Verification items for the finished model (mm, model axes). Face numbers are marked on the shaded views. A direction names the side the tool comes from. Give positions to 0.01 mm unless a question says otherwise; leave off trailing zeros. Order: outer loops, then holes, each group sorted by start corner. A loop starts at its lowest first (then second) coordinate and runs counter-clockwise, first axis right, second up.
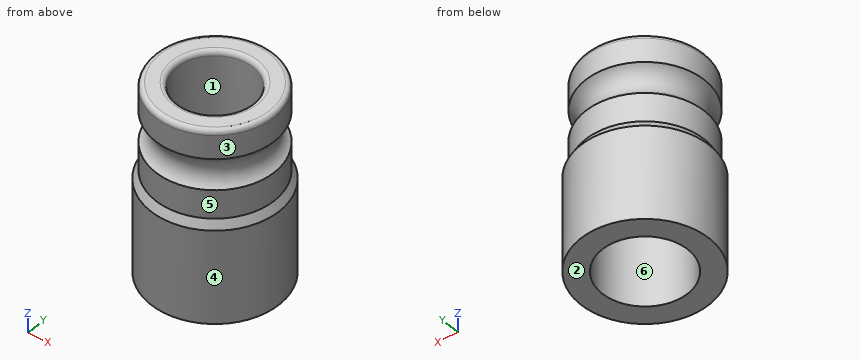
from build123d import *

# Parameters (mm, degrees)
F2_R     = 2
F3_R     = 18
F3_R_2   = 14
F4_DEPTH = 30


# Not quite as in the source:
# - a feature names something its author has since deleted; it is built from what else it names


with BuildPart() as f1:
    # F0 (on Front) → F1 (revolve)
    with BuildSketch(Plane.XZ):
        with BuildLine():
            Line((-14, -9.4360596032), (-16, 40.5639403968))
            Line((-16, 40.5639403968), (-25, 40.5639403968))
            Line((-25, 40.5639403968), (-25, 28.5639403968))
            ThreePointArc((-25, 28.5639403968), (-21.593316446, 22.014021006), (-25, 15.4641016151))
            Line((-25, 15.4641016151), (-25, 3.4641016151))
            Line((-25, 3.4641016151), (-27, 0))
            Line((-27, 0), (-27, -39.4360596032))
            Line((-27, -39.4360596032), (-18, -39.4360596032))
            Line((-18, -39.4360596032), (-14, -39.4360596032))
            Line((-14, -39.4360596032), (-14, -9.4360596032))
        make_face()
    revolve(axis=Axis((0, 0, -1.7232764512), (0, 0, -1)))

    # F2
    f2_edges = [f1.edges().sort_by_distance(p)[0] for p in [
        (16, 0, 40.56394),
        (25, 0, 40.56394),
    ]]
    fillet(f2_edges, radius=F2_R)

    # F3 (on face) → F4 (cut)
    with BuildSketch(Plane(origin=(0, 0, -39.4360596032), x_dir=(1, 0, 0), z_dir=(0, 0, -1))):
        Circle(F3_R)
        Circle(F3_R_2, mode=Mode.SUBTRACT)
    extrude(amount=-F4_DEPTH, mode=Mode.SUBTRACT)


solid = f1.part
(1) Set-up check for the marked faces 4, 5 and 6: record each of +Z, -Z, +X, -X, +Y, -Y from which the full face is reachable in a straight line by a thin tool's end or side.
Solved:
face 4: +Z, -Z
face 5: +Z
face 6: -Z
(2) Go/stop test with flat-tipped pins: pin 1 (1 mm diameter, centred on x = 4.5, z = -21.5, fed in from -Y); pin 2 (8 mm diameter, centred on x = -5.5, z = 28, fed in from -Y); pin 3 (11 mm diameter, centred on x = 3.5, y = 2, fed in from -Z); pin 4 (4 mm diameter, centred on x = 9, z = -0.5, fed in from +Y). Record where each tip stops, or that it passes through.
Solved:
pin 1: stops at y = -26.7
pin 2: stops at y = -24.95
pin 3: passes through
pin 4: stops at y = 26.08
(3) Section check A-A, the plane x = 0. Enter the section's corners in (y, z).
Solved:
outline: (-27, -39.44) - (-18, -39.44) - (-18, -9.44) - (-14, -9.44) - (-15.92, 38.64) arc R2 ccw to (-17.92, 40.56) - (-23, 40.56) arc R2 ccw to (-25, 38.56) - (-25, 28.56) arc R8 cw to (-25, 15.46) - (-25, 3.46) - (-27, 0) - close; (14, -9.44) - (18, -9.44) - (18, -39.44) - (27, -39.44) - (27, 0) - (25, 3.46) - (25, 15.46) arc R8 cw to (25, 28.56) - (25, 38.56) arc R2 ccw to (23, 40.56) - (17.92, 40.56) arc R2 ccw to (15.92, 38.64) - close
(4) Section check C-C, the plane z = -22. Enter the section's corners in (x, y), then the cut area to 3 significant figures.
Solved:
outline: circle Ø54 at (0, 0); hole circle Ø36 at (0, 0)
area: 1,270 mm2
(5) Release check for a two-part mould opening along Y. For the marked faces 1, 2 and 3 record: pulls with the +Y half, pulls with the -Y half, needs draft (parallel to the pull), parting line crosses it, or undercut.
Solved:
face 1: undercut
face 2: needs draft
face 3: parting line crosses it
(6) Section check D-D, the plane z = 25.5. Enter the section's corners in (x, y), then the cut area to 3 significant figures.
Solved:
outline: circle Ø44.79 at (0, 0); hole circle Ø30.79 at (0, 0)
area: 830 mm2
(7) Scan lines: line 1 (Y direction, x = 0, z = -18); line 2 (X direction, y = 13.5, z = -28); line 3 (Y direction, x = -10, z = 34). Record each from-to range of solid material in increasing order.
Solved:
line 1: y = -27 to -18, 18 to 27
line 2: x = -23.38 to -11.91, 11.91 to 23.38
line 3: y = -22.91 to -12.15, 12.15 to 22.91
